Part model, mm, in its own coordinate system. Face numbers are marked on the shaded views. Coordinates: 2 decimals unless noted, no trailing zeros. Loops run counter-clockwise (first coordinate to the right, second up) from the corner with the lowest first, then second, coordinate; pieces in that order, holes last. Notation, with made-up numbers: (17, -34.5) - (35, -34.5) arc R11 ccw to (35, -17.5) - close; hole circle Ø10 at (-22, 18). An arc over 180 degrees is marked (long way). Use a Markdown table: item, result. Add a question column.
1) Band-saw the part on C-C (z = 25). Give the cut face in (x, y).
2) Probe probe 1 along X at (y, z) = (-6.5, -2.5); probe 2 along X at (y, z) = (-11.25, -1); probe 3 along Y at (x, z) = (71, 29). List the from-to ranges inside material, lowest first. Write a range as [from, to].
3) Band-saw the part on B-B (x = -29). Give the cut face in (y, z), plus the area to 3 significant figures.
4) Band-saw the part on A-A (z = 4.5). Give the cut face in (x, y).
5) Pull direction X, two halves, no side cores. Call the marked faces 1, 2, 3 and 4: +X half, -X half, draft (parallel to the pull), parting line (faces both ways), or undercut.
6) Drop flat-ended pins along their axis: P1, Ø2.5, axis at x = -82, y = -10, coming from the +Z side; P2, Ø1.2, axis at x = -7, y = -12, coming from the +Z side; P3, Ø6, axis at x = -5.5, y = -7, coming from the +Z side. Give the stop position or say it passes through.
from build123d import *

# Parameters (mm, degrees)
F0_W     = 170
F0_H     = 35
F1_DEPTH = 15
F2_W     = 162
F2_H     = 7.2
F3_DEPTH = 32
F4_W     = 170
F4_H     = 3.9
F5_DEPTH = 25
F6_W     = 150
F6_H     = 28.3669353649
F7_DEPTH = 6.3
F8_R     = 5


with BuildPart() as f1:
    # F0 (on Front) → F1 (new body)
    with BuildSketch(Plane.XZ):
        Rectangle(F0_W, F0_H)
    extrude(amount=F1_DEPTH)

    # F2 (on face) → F3 (cut)
    with BuildSketch(Plane.XY.offset(17.5)):
        with Locations((0, -7.5)):
            Rectangle(F2_W, F2_H)
    extrude(amount=-F3_DEPTH, mode=Mode.SUBTRACT)

    # F4 (on face) → F5 (join)
    with BuildSketch(Plane.XY.offset(17.5)):
        with Locations((0, -1.95)):
            Rectangle(F4_W, F4_H)
    extrude(amount=F5_DEPTH)

    # F6 (on face) → F7 (cut)
    with BuildSketch(Plane.XZ.offset(15)):
        with Locations((0, 3.3165323175)):
            Rectangle(F6_W, F6_H)
    extrude(amount=-F7_DEPTH, mode=Mode.SUBTRACT)

    # F8
    f8_edges = [f1.edges().sort_by_distance(p)[0] for p in [
        (-85, -1.95, 42.5),
        (85, -1.95, 42.5),
        (75, -13.05, 17.5),
        (-75, -13.05, 17.5),
    ]]
    fillet(f8_edges, radius=F8_R)


solid = f1.part
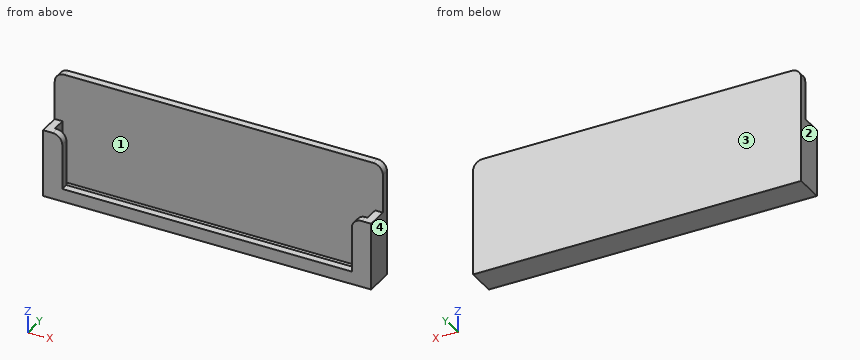
Answer block:
| question | item | result |
|---|---|---|
| 1 | outline | (-85, -3.9) - (85, -3.9) - (85, 0) - (-85, 0) - close |
| 2 | probe 1 | [-85, -81], [81, 85] |
| 2 | probe 2 | [-85, -75], [75, 85] |
| 2 | probe 3 | [-3.9, 0] |
| 3 | outline | (-15, -17.5) - (0, -17.5) - (0, 42.5) - (-3.9, 42.5) - (-3.9, -14.5) - (-11.1, -14.5) - (-11.1, -10.87) - (-15, -10.87) - close |
| 3 | area | 281 mm2 |
| 4 | outline | (-85, -15) - (-75, -15) - (-75, -11.1) - (-81, -11.1) - (-81, -3.9) - (81, -3.9) - (81, -11.1) - (75, -11.1) - (75, -15) - (85, -15) - (85, 0) - (-85, 0) - close |
| 5 | face 1 | undercut |
| 5 | face 2 | -X half |
| 5 | face 3 | draft |
| 5 | face 4 | +X half |
| 6 | P1 | z = 17.5 |
| 6 | P2 | z = -10.87 |
| 6 | P3 | z = -14.5 |
